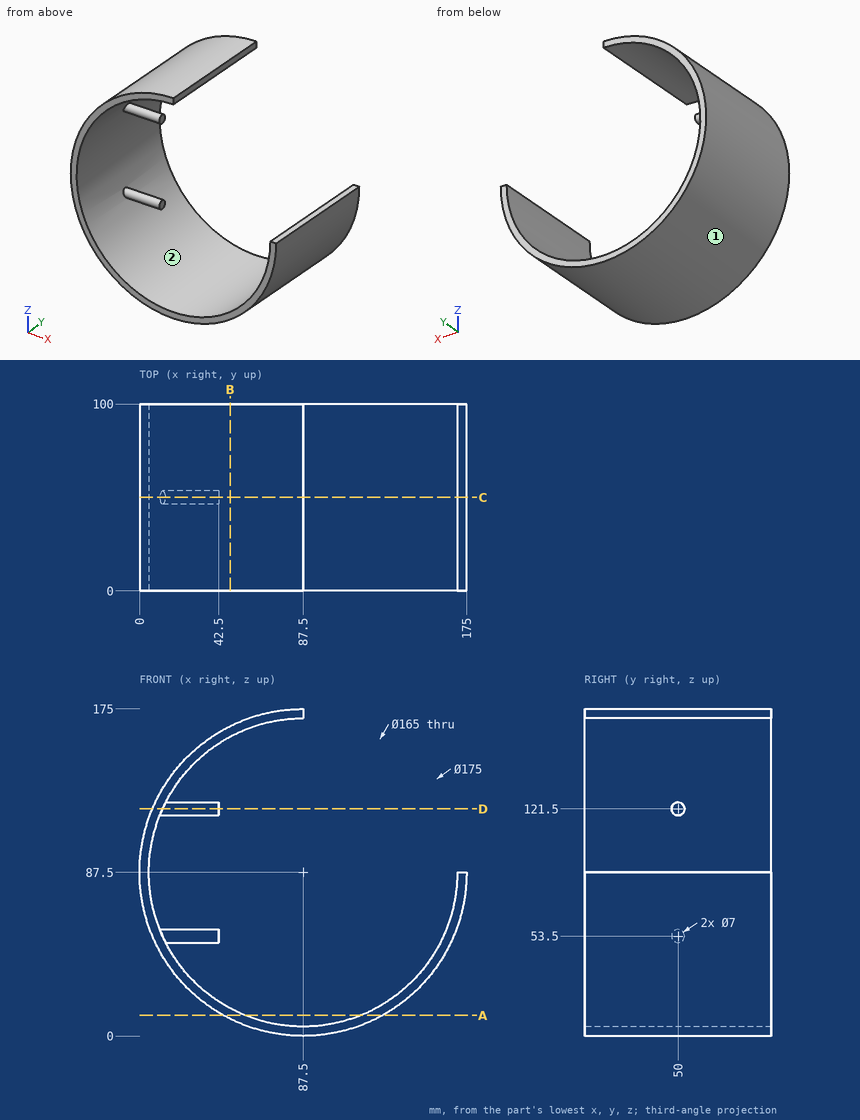
Answer from the drawing. Dimensions are ordinates in mm from the lowest x, y and z of the part. Round coordinates to 2 decimals unless told otherwise and drop trailing zeros. Write each loop counter-clockwise with the first axis right and the second up, starting at its lowest first coordinate (ties: lowest second). Pieces come first, ordered by that corner, then holes. Notation, with made-up numbers: (80.25, -21.75) -> (90.25, -21.75) arc R29 ccw to (90.25, 14.25) -> close; hole circle Ø3 at (84, 79.5). An arc over 180 degrees is marked (long way). Answer in a Markdown table with one row per item. Add a question column.
1) Given P1, Ø2, axis at y = 35.5, z = 54, coming from the +X side; P2, Ø2, axis at y = 51.5, z = 122, coming from the +X side; P3, Ø8, axis at y = 77, z = 127, coming from the +X side, each flat-ended and moving along its own axis, determine where each tip first touches the part or whether it passes through.
2) Find section A-A, the plane z = 11. Determine the outline of the cut face in (x, y).
3) Find section C-C, the plane y = 50. Determine the outline of the cut face in (x, z), and give its area (3 significant figures).
4) Determine the mould class of the marked faces 1 and 2 for opening direction X: pulls with the +X half, pulls with the -X half, needs draft (parallel to the pull), parting line crosses it, or undercut.
5) Find section B-B, the plane x = 48.5. Determine the outline of the cut face in (y, z).
6) Find section D-D, the plane z = 121.5. Determine the outline of the cut face in (x, y).
7) Consider line 1 (Z direction, x = 87, y = 27); line 2 (Z direction, x = 11, y = 64); line 3 (X direction, y = 30, z = 32). Determine where each line is inside the solid, lowest interval first.
Findings below:
| question | item | result |
|---|---|---|
| 1 | P1 | x = 168.74 |
| 1 | P2 | x = 42.5 |
| 1 | P3 | x = 17.4 |
| 2 | outline | (45.03, 0) -> (56.61, 0) -> (56.61, 100) -> (45.03, 100) -> close; (118.39, 0) -> (129.97, 0) -> (129.97, 100) -> (118.39, 100) -> close |
| 3 | outline | (10.84, 57) arc R82.5 cw to (10.84, 118) -> (42.5, 118) -> (42.5, 125) -> (14.02, 125) arc R82.5 cw to (87.5, 170) -> (87.5, 175) arc R87.5 ccw (long way) to (175, 87.5) -> (170, 87.5) arc R82.5 cw to (14.02, 50) -> (42.5, 50) -> (42.5, 57) -> close |
| 3 | area | 2,420 mm² |
| 4 | face 1 | parting line crosses it |
| 4 | face 2 | undercut |
| 5 | outline | (0, 9.17) -> (100, 9.17) -> (100, 14.8) -> (0, 14.8) -> close; (0, 160.2) -> (100, 160.2) -> (100, 165.83) -> (0, 165.83) -> close |
| 6 | outline | (6.88, 0) -> (12.33, 0) -> (12.33, 46.5) -> (42.5, 46.5) -> (42.5, 53.5) -> (12.33, 53.5) -> (12.33, 100) -> (6.88, 100) -> close |
| 7 | line 1 | 0 to 5, 170 to 175 |
| 7 | line 2 | 45.03 to 56.61, 118.39 to 129.97 |
| 7 | line 3 | 19.85 to 26.46, 148.54 to 155.15 |
